Can you work these out from the model? Positions are in its coordinate system, mm. A direction names the side the tool comes from. Coordinates: 2 decimals unless noted, no trailing zeros. Order: outer loops, then holes, each group sorted by start corner. A loop starts at its lowest first (then second) coordinate and runs counter-clockwise, first axis right, second up.
```python
from build123d import *

# Parameters (mm, degrees)
F0_W     = 50.8
F0_H     = 38.1
F1_DEPTH = 2.54
F2_W     = 46.99
F2_H     = 38.1
F3_DEPTH = 2.54
F4_R     = 1.905
F5_DEPTH = 38.101


with BuildPart() as f1:
    # F0 (on Top) → F1 (new body)
    with BuildSketch(Plane.XY):
        Rectangle(F0_W, F0_H)
    extrude(amount=F1_DEPTH)

    # F2 (on face) → F3 (join)
    with BuildSketch(Plane.XZ.offset(19.05)):
        with Locations((0, -16.51)):
            Rectangle(F2_W, F2_H)
    extrude(amount=F3_DEPTH)

    # F4 (on face) → F5 (cut, through all)
    with BuildSketch(Plane.XY.offset(2.54)):
        with Locations((20.6375, 13.97)):
            Circle(F4_R)
        with Locations((-20.6375, 13.97)):
            Circle(F4_R)
    extrude(amount=-F5_DEPTH, mode=Mode.SUBTRACT)


solid = f1.part
```
1. Imagine slicing it at B-B on x = 13.5. Please give me the cut outline in (y, z).
Completed:
outline: (-21.59, -35.56) - (-19.05, -35.56) - (-19.05, 0) - (19.05, 0) - (19.05, 2.54) - (-21.59, 2.54) - close
2. I'm going to push flat-ended pins straight in: pin 1 (3 mm diameter, centred on y = -20, z = -18.5, fed in from +X) (3 decimals); pin 2 (10.5 mm diameter, centred on x = 11, z = -26.5, fed in from +Y); pin 3 (5 mm diameter, centred on x = 12.5, y = -6, fed in from -Z). Where does each tip first touch, or does it pass through?
Completed:
pin 1: stops at x = 23.495
pin 2: stops at y = -19.05
pin 3: stops at z = 0
3. On a 3-axis mill with a long thin cutter (end or side, diameter ignored), from which of +Z, -Z, +X, -X, +Y, -Y can I reach the whole of each face in a straight line? I mean faces 4 (the flat face through (0, -1, 2.54)), 5 (the flat face through (0, -19.05, -18)), 6 (the flat face through (24, -19.05, 1)). Say none if no direction works.
Completed:
face 4: +Z, +X, -X, +Y, -Y
face 5: -Z, +X, -X, +Y
face 6: +Z, -Z, +X, -Y
4. Thinking about a two-plate mould opening in Y: for faces 1 (the flat face through (-24, -19.05, 1)), 2 (the flat face through (23.495, -20, -17)), 3 (the cylindrical face through (-22.54, 14.05, 1.29)), which applies, pulls with the +Y half, pulls with the -Y half, needs draft (parallel to the pull), parting line crosses it, or undercut?
Completed:
face 1: pulls with the -Y half
face 2: needs draft
face 3: undercut
5. Please list where these lines run through material, in increasing order: probe 1 along Z at (x, y) = (-10.5, -4); probe 2 along Y at (x, z) = (22.5, -18); probe 3 along X at (y, z) = (-19.5, -16.5) (3 decimals).
Completed:
probe 1: z = 0 to 2.54
probe 2: y = -21.59 to -19.05
probe 3: x = -23.495 to 23.495
6. Imagine slicing it at C-C on y = 0. Please give me the cut outline in (x, z), then the cut area to 3 significant figures.
Completed:
outline: (-25.4, 0) - (25.4, 0) - (25.4, 2.54) - (-25.4, 2.54) - close
area: 129 mm2
7. Imagine slicing it at D-D on z = -7. Please give me the cut outline in (x, y) (3 decimals).
Completed:
outline: (-23.495, -21.59) - (23.495, -21.59) - (23.495, -19.05) - (-23.495, -19.05) - close
8. Imagine slicing it at A-A on y = 13.97. Please give me the cut outline in (x, z).
Completed:
outline: (-25.4, 0) - (-22.54, 0) - (-22.54, 2.54) - (-25.4, 2.54) - close; (-18.73, 0) - (18.73, 0) - (18.73, 2.54) - (-18.73, 2.54) - close; (22.54, 0) - (25.4, 0) - (25.4, 2.54) - (22.54, 2.54) - close
